Input: part model. Units: mm. Frame: model coordinates. Face numbers are marked on the shaded views. A direction names the side the tool comes from. Coordinates: 2 decimals unless noted, no trailing zeros. Write each loop counter-clockwise with the first axis right and the second up, starting at its lowest first coordinate (ties: lowest second). Pieces come first, ordered by that corner, then holes. Notation, with made-up numbers: M 72,71.25 L 90,71.25 A21 cw 90,102.25 Z; hole C 49.5,15.5 d10. An arc over 180 degrees is marked long. Use one line per item in the form item = value.
from build123d import *

# Parameters (mm, degrees)
F0_R            = 50
F1_DEPTH        = 8
F2_R            = 20
F3_DEPTH        = 35
F5_D            = 4
F5_DEPTH        = 12
F5_CBORE_D      = 8
F5_CBORE_DEPTH  = 3
F5_TIP          = 1.2017212381
F5_COPIES_COUNT = 5
F6_SIZE         = 1.5
F7_R            = 15
F8_DEPTH        = 43.001
F9_SIZE         = 1
F10_SIZE        = 1


# Not quite as in the source:
# - a pattern or mirror of a feature is missing from the dataset's text; its kind, count and spacing are read off the source's solid


with BuildPart() as f1:
    # F0 (on Top) → F1 (new body)
    with BuildSketch(Plane.XY):
        Circle(F0_R)
    extrude(amount=F1_DEPTH)

    # F2 (on face) → F3 (join)
    with BuildSketch(Plane.XY.offset(8)):
        Circle(F2_R)
    extrude(amount=F3_DEPTH)

    # F5
    with Locations(Plane.XY.offset(8)):
        with Locations((34.9212251604, 7.7109653503)):
            f5 = CounterBoreHole(F5_D / 2, F5_CBORE_D / 2, F5_CBORE_DEPTH, depth=F5_DEPTH)
            with Locations((0, 0, -(F5_DEPTH + F5_TIP / 2))):  # 118° drill point
                Cone(0, F5_D / 2, F5_TIP, mode=Mode.SUBTRACT)

    # F5_copies: F5 ×5 about axis
    f5_copies_axis = Axis((0, 0, 0), (0, 0, 1))
    for i in range(1, F5_COPIES_COUNT):
        add(f5.rotate(f5_copies_axis, i * 360 / F5_COPIES_COUNT), mode=Mode.SUBTRACT)

    # F6
    f6_edges = [f1.edges().sort_by_distance(p)[0] for p in [
        (-20, 0, 43),
    ]]
    chamfer(f6_edges, length=F6_SIZE)

    # F7 (on face) → F8 (cut, through all)
    with BuildSketch(Plane.XY.offset(43)):
        Circle(F7_R)
    extrude(amount=-F8_DEPTH, mode=Mode.SUBTRACT)

    # F9
    f9_edges = [f1.edges().sort_by_distance(p)[0] for p in [
        (-50, 0, 8),
        (-50, 0, 0),
    ]]
    chamfer(f9_edges, length=F9_SIZE)

    # F10
    f10_edges = [f1.edges().sort_by_distance(p)[0] for p in [
        (-15, 0, 0),
    ]]
    chamfer(f10_edges, length=F10_SIZE)


solid = f1.part
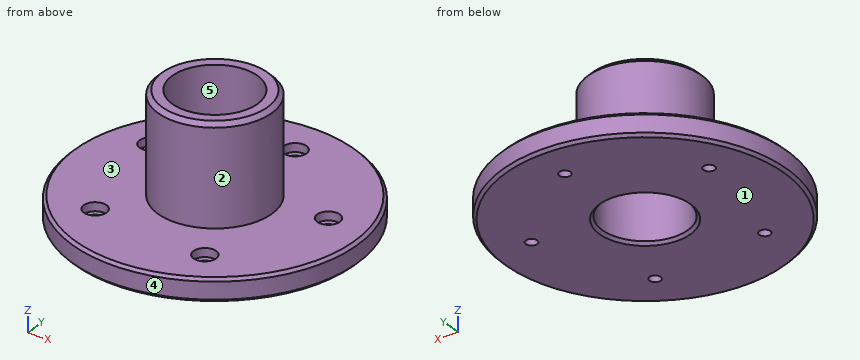
(1) Set-up query: the marked faces 1 and 2. Return all of +Z, -Z, +X, -X, +Y, -Y with unobstructed straight access to the full face (end or side cutting, diameter ignored); none if empty.
Computed:
face_1 = -Z, +X, -X, +Y, -Y
face_2 = +Z
(2) Section query A-A on y = 0. Return the cut outline in (x, z), plus the area to 3 significant figures.
Computed:
outline = M -50,1 L -49,0 L -16,0 L -15,1 L -15,43 L -18.5,43 L -20,41.5 L -20,8 L -49,8 L -50,7 Z; M 15,1 L 16,0 L 49,0 L 50,1 L 50,7 L 49,8 L 20,8 L 20,41.5 L 18.5,43 L 15,43 Z
area = 905 mm^2
(3) Pull-direction query (Y, two-part tool) for the marked faces 3, 4 and 5; classes: pulls with the +Y half, pulls with the -Y half, needs draft (parallel to the pull), parting line crosses it, or undercut.
Computed:
face_3 = needs draft
face_4 = parting line crosses it
face_5 = undercut
(4) First-contact query: pin 1 Ø9 at (x, y) = (36, 9.5) entering from +Z; pin 2 Ø5 at (x, y) = (3.46, 35.59) entering from +Z; pin 3 Ø8 at (x, z) = (-38, 5.5) entering from +Y. Flat tips, straight axial feed; report the tip coordinate or a pass-through.
Computed:
pin_1 = 8
pin_2 = 5
pin_3 = 36.66
(5) Line query: probe 1 along Z at (x, y) = (-27, -18.5); probe 2 along Y at (x, z) = (0.5, 14.5); probe 3 along Y at (x, z) = (-4, 16). Output: solid intervals per line, ascending.
Computed:
probe_1 = 0 to 8
probe_2 = -19.99 to -14.99, 14.99 to 19.99
probe_3 = -19.6 to -14.46, 14.46 to 19.6
(6) Section query B-B on z = 19. Return the cut outline in (x, y).
Computed:
outline = C 0,0 d40; hole C 0,0 d30
